Geometry check sheet. Reference: drawing and pictorial views, mm from the part's lowest x, y, z. A direction names the side the tool comes from. Round coordinates to 2 decimals unless told otherwise and drop trailing zeros. Order: outer loops, then holes, each group sorted by start corner. A loop starts at its lowest first (then second) coordinate and runs counter-clockwise, first axis right, second up.
(1) Go/stop test with flat-tipped pins: pin 1 (8 mm diameter, centred on x = 26.5, z = 65.5, fed in from +Y); pin 2 (5 mm diameter, centred on x = 15.5, z = 84, fed in from -Y); pin 3 (10 mm diameter, centred on y = 76, z = 32.5, fed in from -X). Record where each tip stops, or that it passes through.
(2) Sectioned sample at C-C (y = 5). Record the boundary of the cut face in (x, z) (3 decimals), plus the area to 3 significant figures.
(3) Material ranges on line 1 along Y through (x, z) = (40, 5); line 2 along Y through (x, z) = (40, 42); line 3 along Z through (x, y) = (28, 67), recorded low to high.
(4) Sectioned sample at B-B (z = 94). Record the boundary of the cut face in (x, y), plus the area to 3 significant figures.
(5) Release check for a two-part mould opening along X. For the marked faces 3, 4 and 5 record: +X half, -X half, draft (parallel to the pull), parting line (faces both ways), or undercut.
(6) Sectioned sample at D-D (y = 22.5). Record the boundary of the cut face in (x, z), plus the area to 3 significant figures.
(7) Sectioned sample at A-A (x = 40). Record the boundary of the cut face in (y, z), plus the area to 4 significant figures.
(8) Set-up check for the marked faces 1 and 2: record each of +Z, -Z, +X, -X, +Y, -Y from which the full face is reachable in a straight line by a thin tool's end or side.
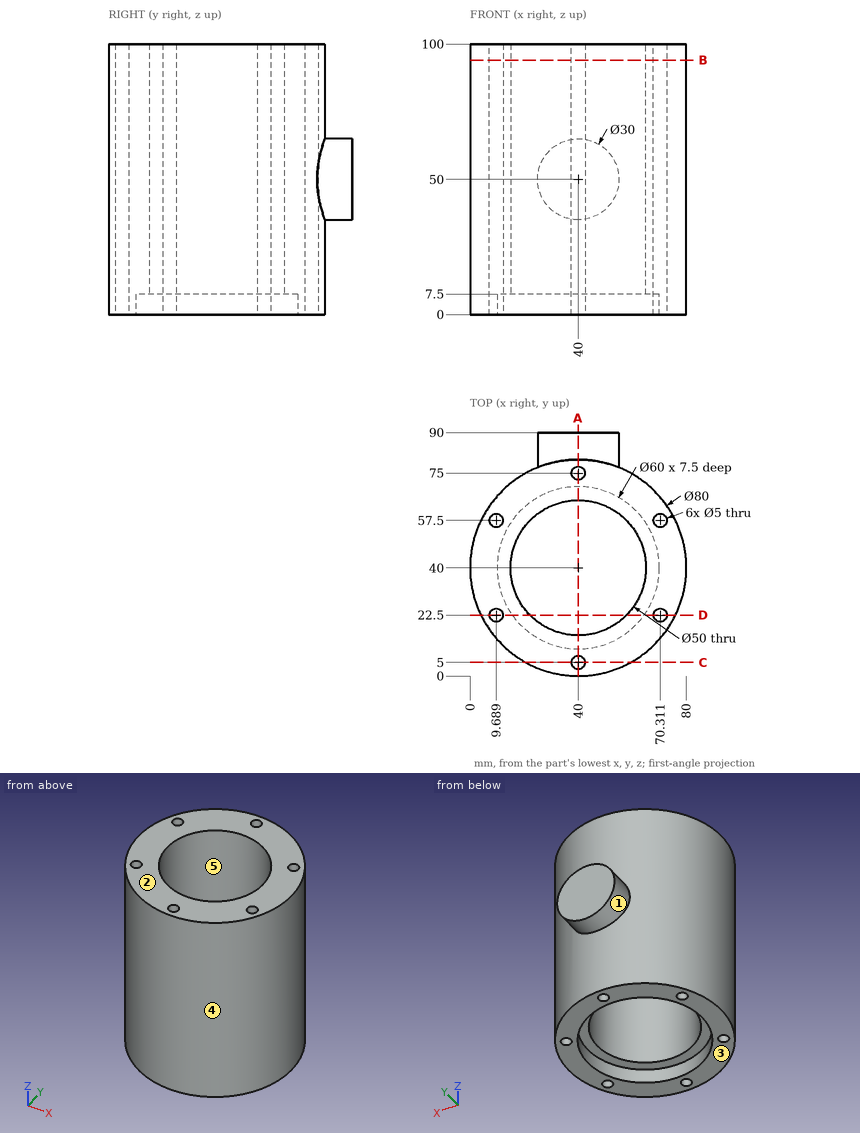
Answer below:
1. pin 1: stops at y = 78.86
1. pin 2: stops at y = 6.59
1. pin 3: stops at x = 14.72
2. outline: (20.635, 0) - (37.5, 0) - (37.5, 100) - (20.635, 100) - close; (42.5, 0) - (59.365, 0) - (59.365, 100) - (42.5, 100) - close
2. area: 3,370 mm2
3. line 1: y = 0 to 2.5, 7.5 to 10, 70 to 72.5, 77.5 to 80
3. line 2: y = 0 to 2.5, 7.5 to 15, 65 to 72.5, 77.5 to 90
3. line 3: z = 7.5 to 100
4. outline: circle Ø80 at (40, 40); hole circle Ø5 at (9.69, 22.5); hole circle Ø5 at (9.69, 57.5); hole circle Ø50 at (40, 40); hole circle Ø5 at (40, 5); hole circle Ø5 at (40, 75); hole circle Ø5 at (70.31, 22.5); hole circle Ø5 at (70.31, 57.5)
4. area: 2,950 mm2
5. face 3: draft
5. face 4: parting line
5. face 5: undercut
6. outline: (4.03, 0) - (7.19, 0) - (7.19, 100) - (4.03, 100) - close; (12.19, 0) - (15.63, 0) - (15.63, 7.5) - (22.15, 7.5) - (22.15, 100) - (12.19, 100) - close; (57.85, 7.5) - (64.37, 7.5) - (64.37, 0) - (67.81, 0) - (67.81, 100) - (57.85, 100) - close; (72.81, 0) - (75.97, 0) - (75.97, 100) - (72.81, 100) - close
6. area: 2,530 mm2
7. outline: (0, 0) - (2.5, 0) - (2.5, 100) - (0, 100) - close; (7.5, 0) - (10, 0) - (10, 7.5) - (15, 7.5) - (15, 100) - (7.5, 100) - close; (65, 7.5) - (70, 7.5) - (70, 0) - (72.5, 0) - (72.5, 100) - (65, 100) - close; (77.5, 0) - (80, 0) - (80, 35) - (90, 35) - (90, 65) - (80, 65) - (80, 100) - (77.5, 100) - close
7. area: 2,225 mm2
8. face 1: +Y
8. face 2: +Z, +X, -X, +Y, -Y
